Can you work these out from the model? Positions are in its coordinate system, mm. A direction names the side the tool comes from. Round coordinates to 2 decimals unless told otherwise and drop trailing zeros. Order: outer loops, then holes, each group sorted by start corner. A loop starts at its lowest first (then second) coordinate and runs counter-clockwise, first axis right, second up. Notation, with made-up numbers: M 75,4 L 91,4 A33 ccw 91,42 Z; hole C 36.25,59.25 d5. An arc over 180 degrees is marked long. One line per question, with ' | ' between items.
```python
from build123d import *

# Parameters (mm, degrees)
F0_W      = 25.4
F0_H      = 38.1
F1_DEPTH  = 25.4
F3_DEPTH  = 50.8
F4_W      = 12.7
F4_H      = 19.05
F5_DEPTH  = 50.8
F7_W      = 12.7
F7_H      = 6.35
F8_DEPTH  = 25.4
F9_W      = 8.128
F9_H      = 6.35
F10_DEPTH = 25.4


with BuildPart() as f1:
    # F0 (on Top) → F1 (new body)
    with BuildSketch(Plane.XY):
        with Locations((12.7, 19.05)):
            Rectangle(F0_W, F0_H)
    extrude(amount=F1_DEPTH)

    # F2 (on Front) → F3 (cut)
    with BuildSketch(Plane.XZ):
        Polygon((25.4, 25.4), (0, 25.4), (25.4, 6.35), align=None)
    extrude(amount=-F3_DEPTH, mode=Mode.SUBTRACT)

    # F4 (on Right) → F5 (cut)
    with BuildSketch(Plane.YZ):
        with Locations((6.35, 15.875)):
            Rectangle(F4_W, F4_H)
    extrude(amount=F5_DEPTH, mode=Mode.SUBTRACT)

    # F7 (on Right) → F8 (cut)
    with BuildSketch(Plane.YZ):
        with Locations((19.05, 22.225)):
            Rectangle(F7_W, F7_H)
    extrude(amount=F8_DEPTH, mode=Mode.SUBTRACT)

    # F9 (on Front) → F10 (cut)
    with BuildSketch(Plane.XZ):
        with Locations((21.336, 9.525)):
            Rectangle(F9_W, F9_H)
    extrude(amount=-F10_DEPTH, mode=Mode.SUBTRACT)


solid = f1.part
```
(1) If we section it at B-B on y = 24: Please give me the cut outline in (x, z).
Final values:
outline: M 0,0 L 25.4,0 L 25.4,6.35 L 17.27,6.35 L 17.27,12.45 L 8.47,19.05 L 0,19.05 Z
(2) Please list where these lines run through material, in increasing order: probe 1 along Y at (x, z) = (7.75, 15.75); probe 2 along Z at (x, y) = (24, 21.5); probe 3 along X at (y, z) = (14.5, 12). Write a range as [from, to].
Final values:
probe 1: [12.7, 38.1] | probe 2: [0, 6.35] | probe 3: [0, 17.27]
(3) Will these pins go through, and if not, where does the flat tip stop? pin 1 Ø1.5 at (y, z) = (26, 17) entering from +X; pin 2 Ø5 at (y, z) = (22, 10.5) entering from +X; pin 3 Ø7.5 at (x, y) = (14, 16) entering from +Z.
Final values:
pin 1: x = 12.2 | pin 2: x = 17.27 | pin 3: z = 17.71
(4) If we section it at A-A on x = 15: Please give me the cut outline in (y, z).
Final values:
outline: M 0,0 L 38.1,0 L 38.1,14.15 L 12.7,14.15 L 12.7,6.35 L 0,6.35 Z
(5) If we section it at D-D on z = 16.5: Please give me the cut outline in (x, y), plus the area to 3 significant figures.
Final values:
outline: M 0,12.7 L 11.87,12.7 L 11.87,38.1 L 0,38.1 Z | area: 301 mm^2
(6) If we section it at C-C on x = 10: Please give me the cut outline in (y, z), plus the area to 3 significant figures.
Final values:
outline: M 0,0 L 38.1,0 L 38.1,17.9 L 12.7,17.9 L 12.7,6.35 L 0,6.35 Z | area: 535 mm^2
(7) On a 3-axis mill with a long thin cutter (end or side, diameter ignored), from which of +Z, -Z, +X, -X, +Y, -Y can I reach the whole of each face in a straight line? I mean faces 1 (the flat face through (25.4, 19, 3)), 2 (the flat face through (19, 25.4, 8)), 3 (the flat face through (3, 25.4, 21)). Say none if no direction works.
Final values:
face 1: +Z, -Z, +X, +Y, -Y | face 2: +Z, +X, -Y | face 3: +Z, +X, -X, -Y
